```python
from build123d import *

# Parameters (mm, degrees)
BOSS_EXTRUDE1_DEPTH = 76.2
SKETCH2_R           = 12.7
BOSS_EXTRUDE2_DEPTH = 50.8


with BuildPart() as part:
    # Sketch1 → Boss-Extrude1 (new body, symmetric)
    with BuildSketch(Plane(origin=(0, 0, 0), x_dir=(0, 0, -1), z_dir=(1, 0, 0))):
        with BuildLine():
            Line((-53.5, 63.5), (53.5, 63.5))
            ThreePointArc((53.5, 63.5), (60.571067812, 60.571067812), (63.5, 53.5))
            Line((63.5, 53.5), (63.5, -53.5))
            ThreePointArc((63.5, -53.5), (60.571067812, -60.571067812), (53.5, -63.5))
            Line((53.5, -63.5), (-53.5, -63.5))
            ThreePointArc((-53.5, -63.5), (-60.571067812, -60.571067812), (-63.5, -53.5))
            Line((-63.5, -53.5), (-63.5, 53.5))
            ThreePointArc((-63.5, 53.5), (-60.571067812, 60.571067812), (-53.5, 63.5))
        make_face()
    extrude(amount=BOSS_EXTRUDE1_DEPTH, both=True)

    # Sketch2 → Boss-Extrude2 (add)
    with BuildSketch(Plane(origin=(76.2, 0, 0), x_dir=(0, 0, -1), z_dir=(1, 0, 0))):
        Circle(SKETCH2_R)
    extrude(amount=BOSS_EXTRUDE2_DEPTH)


solid = part.part
```
Geometry: final body of the model. Coordinates: model frame, mm. A direction names the side the tool comes from. Give positions to 0.01 mm unless a question says otherwise; leave off trailing zeros. Order: outer loops, then holes, each group sorted by start corner. A loop starts at its lowest first (then second) coordinate and runs counter-clockwise, first axis right, second up. Notation, with made-up numbers: (23.25, 37) -> (62.25, 37) arc R20 cw to (62.25, 49) -> close; hole circle Ø1 at (40, 33). An arc over 180 degrees is marked (long way). Write each question's results on one line, items separated by ' | '. Start each with the question number.
1) Line query: line 1 (X direction, y = -11.5, z = -38); line 2 (Y direction, x = 45, z = 54.5); line 3 (Z direction, x = 100.5, y = 10). Output: solid intervals per line, ascending. Write a range as from..to.
2) Set-up query: faces 1 (the cylindrical face through (101.24, -12.4, 2.75)), 2 (the flat face through (-76.2, 1, -1)). Return all of +Z, -Z, +X, -X, +Y, -Y with unobstructed straight access to the full face (end or side cutting, diameter ignored); none if empty.
3) Section C-C (y = -37). Return loops of the section in (x, z), then the cut area to 3 significant figures.
4) Section A-A (y = 0). Return loops of the section in (x, z), then the cut area to 3 significant figures.
Calculated:
1) line 1: -76.2..76.2 | line 2: -63.45..63.45 | line 3: -7.83..7.83
2) face 1: +X | face 2: +Z, -Z, -X, +Y, -Y
3) outline: (-76.2, -63.5) -> (76.2, -63.5) -> (76.2, 63.5) -> (-76.2, 63.5) -> close | area: 19,400 mm2
4) outline: (-76.2, -63.5) -> (76.2, -63.5) -> (76.2, -12.7) -> (127, -12.7) -> (127, 12.7) -> (76.2, 12.7) -> (76.2, 63.5) -> (-76.2, 63.5) -> close | area: 20,600 mm2
